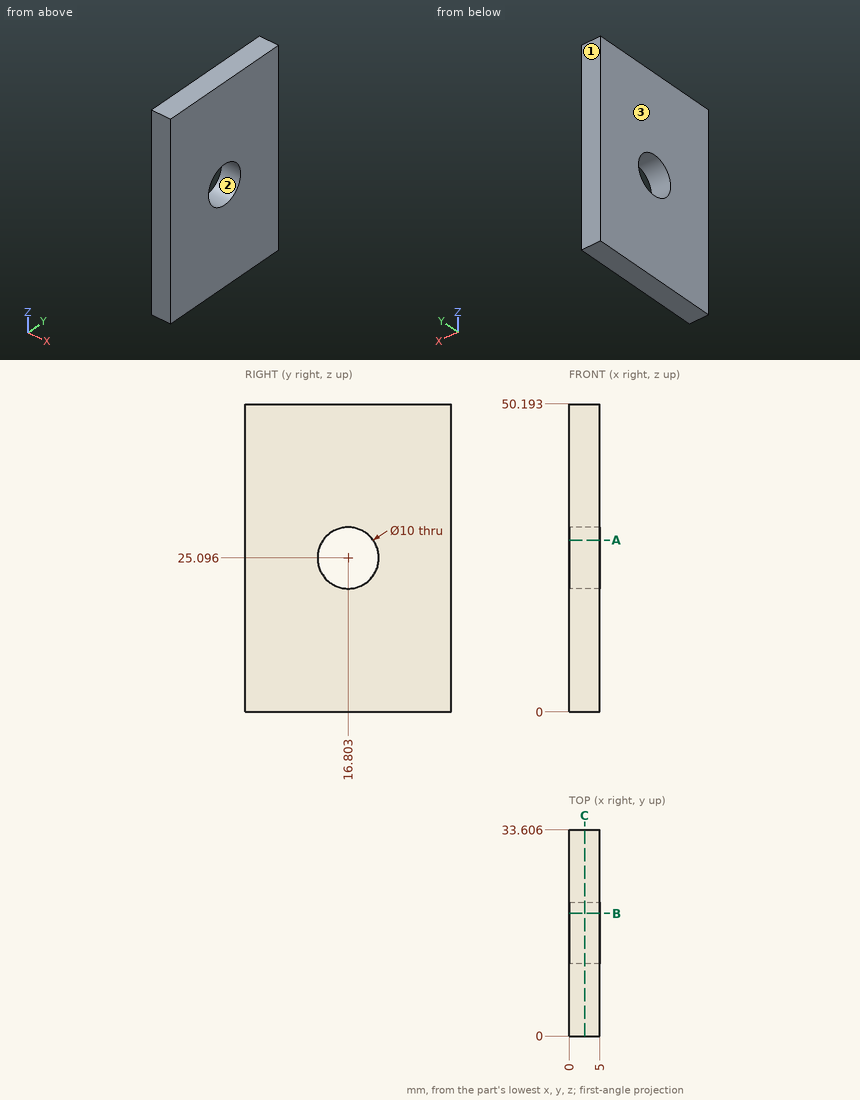
For this review, use the dimensioned drawing (mm, ordinates from the lowest corner) and the shaded views. Coordinates: 2 decimals unless noted, no trailing zeros. Order: outer loops, then holes, each group sorted by start corner. A loop starts at its lowest first (then second) coordinate and runs counter-clockwise, first axis right, second up. Notation, with made-up numbers: (-11.5, -6) - (-3.5, -6) arc R17 cw to (-3.5, 8) - close; hole circle Ø1 at (44, 33). An arc over 180 degrees is marked (long way). Answer as a JSON object with one key per item and string values. Group by question number.
1. We need section C-C on x = 2.5. State the section outline as (y, z) points (1 decimal), then the cut area to 3 significant figures.
2. We need section B-B on y = 20. State the section outline as (x, z) points.
3. We need section A-A on z = 28. State the section outline as (x, y) points (1 decimal), then the cut area to 3 significant figures.
4. For probe 1 along Z at (x, y) = (3.8, 18); probe 2 along Y at (x, z) = (0.9, 24) (1 decimal); probe 3 along Y at (x, z) = (2.1, 25.5) (1 decimal), list the stretches that pass through material, from the lowest coordinate up.
5. The part is to be moulded in two halves that separate along Y. For the marked faces 1, 2 and 3, say which applies: pulls with the +Y half, pulls with the -Y half, needs draft (parallel to the pull), parting line crosses it, or undercut.
Final values:
{
 "1": {"outline": "(0, 0) - (33.6, 0) - (33.6, 50.2) - (0, 50.2) - close; hole circle Ø10 at (16.8, 25.1)", "area": "1,610 mm²"},
 "2": {"outline": "(0, 0) - (5, 0) - (5, 21.25) - (0, 21.25) - close; (0, 28.94) - (5, 28.94) - (5, 50.19) - (0, 50.19) - close"},
 "3": {"outline": "(0, 0) - (5, 0) - (5, 12.7) - (0, 12.7) - close; (0, 20.9) - (5, 20.9) - (5, 33.6) - (0, 33.6) - close", "area": "127 mm²"},
 "4": {"probe 1": "0 to 20.24, 29.95 to 50.19", "probe 2": "0 to 11.9, 21.7 to 33.6", "probe 3": "0 to 11.8, 21.8 to 33.6"},
 "5": {"face 1": "pulls with the +Y half", "face 2": "undercut", "face 3": "needs draft"}
}
